```python
from build123d import *

# Parameters (mm, degrees)
F0_W     = 160.02
F0_H     = 160.02
F1_DEPTH = 29.972
F3_DEPTH = 26.162
F4_R     = 6.35
F4_R_2   = 3.81
F4_R_3   = 3.175
F5_DEPTH = 6.35


with BuildPart() as f1:
    # F0 (on Top) → F1 (new body)
    with BuildSketch(Plane.XY):
        with Locations((80.01, 80.01)):
            Rectangle(F0_W, F0_H)
    extrude(amount=-F1_DEPTH)

    # F2 (on face) → F3 (cut)
    with BuildSketch(Plane(origin=(0, 0, -29.972), x_dir=(1, 0, 0), z_dir=(0, 0, -1))):
        Polygon((18.923, -25.4), (4.445, -25.4), (4.445, -134.62), (18.923, -134.62), (18.923, -155.575), (141.097, -155.575), (141.097, -134.62), (155.575, -134.62), (155.575, -25.4), (141.097, -25.4), (141.097, -4.445), (18.923, -4.445), align=None)
    extrude(amount=-F3_DEPTH, mode=Mode.SUBTRACT)

    # F4 (on face) → F5 (cut)
    with BuildSketch(Plane.XY):
        with Locations((40.005, 38.1)):
            Circle(F4_R)
        with Locations((78.105, 38.1)):
            Circle(F4_R)
        with Locations((116.205, 38.1)):
            Circle(F4_R)
        with Locations((116.205, 76.2)):
            Circle(F4_R_2)
        with Locations((78.105, 76.2)):
            Circle(F4_R_3)
        with Locations((40.005, 76.2)):
            Circle(F4_R_3)
    extrude(amount=-F5_DEPTH, mode=Mode.SUBTRACT)


solid = f1.part
```
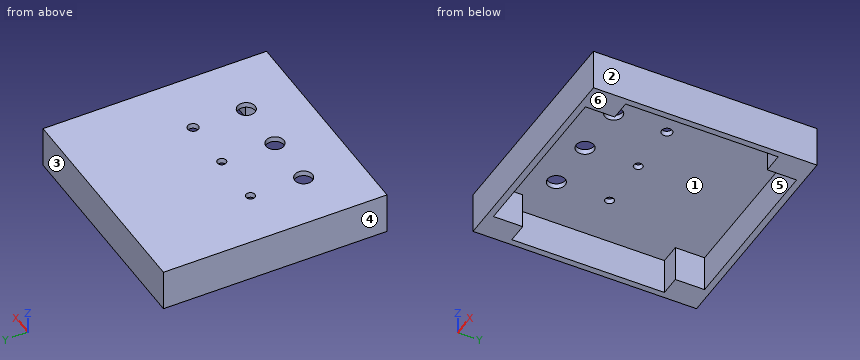
Model file for the job. Use its own axes, mm. Face numbers are marked on the shaded views. A direction names the side the tool comes from. Coordinates: 2 decimals unless noted, no trailing zeros. Write each loop counter-clockwise with the first axis right and the second up, starting at its lowest first coordinate (ties: lowest second). Pieces come first, ordered by that corner, then holes. Notation, with made-up numbers: (74, 65) - (85, 65) arc R16 ccw to (85, 70) - close; hole circle Ø4 at (-28, 22.5). An arc over 180 degrees is marked (long way). Use a Markdown table: item, result. Add a question column.
Item 1: Drop flat-ended pins along their axis: pin 1 (7.5 mm diameter, centred on x = 40.005, y = 76.2, fed in from -Z); pin 2 (6 mm diameter, centred on x = 116.205, y = 76.2, fed in from +Z). Give the stop position or say it passes through.
Item 2: Band-saw the part on B-B, the plane z = -9.75. Write the cut outline in (x, y) (3 decimals).
Item 3: Band-saw the part on D-D, the plane x = 61. Write the cut outline in (y, z) (3 decimals), and give its area (3 significant figures).
Item 4: Band-saw the part on C-C, the plane y = 11.5. Write the cut outline in (x, z).
Item 5: Band-saw the part on A-A, the plane y = 38.1. Write the cut outline in (x, z) (3 decimals), and give its area (3 significant figures).
Item 6: 3-axis set-ups, long thin cutter, end or side, ignore diameter. For the marked faces 5 and 6: which of +Z, -Z, +X, -X, +Y, -Y reach the whole face in a straight line?
Item 7: Two-plate mould, pull along X, no slides. Class the marked faces 1, 2, 3 and 4: pulls with the +X half, pulls with the -X half, needs draft (parallel to the pull), parting line crosses it, or undercut.
Item 8: Drill centre lines: line 1 along X through (y, z) = (107.5, -13.75) (3 decimals); line 2 along Y through (x, z) = (148, -15.5). Where is each one in solid material? Low to high.
A:
| question | item | result |
|---|---|---|
| 1 | pin 1 | stops at z = -3.81 |
| 1 | pin 2 | passes through |
| 2 | outline | (0, 0) - (160.02, 0) - (160.02, 160.02) - (0, 160.02) - close; hole (4.445, 25.4) - (18.923, 25.4) - (18.923, 4.445) - (141.097, 4.445) - (141.097, 25.4) - (155.575, 25.4) - (155.575, 134.62) - (141.097, 134.62) - (141.097, 155.575) - (18.923, 155.575) - (18.923, 134.62) - (4.445, 134.62) - close |
| 3 | outline | (0, -29.972) - (4.445, -29.972) - (4.445, -3.81) - (155.575, -3.81) - (155.575, -29.972) - (160.02, -29.972) - (160.02, 0) - (0, 0) - close |
| 3 | area | 842 mm² |
| 4 | outline | (0, -29.97) - (18.92, -29.97) - (18.92, -3.81) - (141.1, -3.81) - (141.1, -29.97) - (160.02, -29.97) - (160.02, 0) - (0, 0) - close |
| 5 | outline | (0, -29.972) - (4.445, -29.972) - (4.445, -3.81) - (33.655, -3.81) - (33.655, 0) - (0, 0) - close; (46.355, -3.81) - (71.755, -3.81) - (71.755, 0) - (46.355, 0) - close; (84.455, -3.81) - (109.855, -3.81) - (109.855, 0) - (84.455, 0) - close; (122.555, -3.81) - (155.575, -3.81) - (155.575, -29.972) - (160.02, -29.972) - (160.02, 0) - (122.555, 0) - close |
| 5 | area | 697 mm² |
| 6 | face 5 | -Z |
| 6 | face 6 | -Z, +X, -X, +Y, -Y |
| 7 | face 1 | undercut |
| 7 | face 2 | pulls with the +X half |
| 7 | face 3 | needs draft |
| 7 | face 4 | pulls with the -X half |
| 8 | line 1 | x = 0 to 4.445, 155.575 to 160.02 |
| 8 | line 2 | y = 0 to 25.4, 134.62 to 160.02 |
